Model file for the job. Use its own axes, mm. Round coordinates to 2 decimals unless told otherwise and drop trailing zeros. Order: outer loops, then holes, each group sorted by start corner. A loop starts at its lowest first (then second) coordinate and runs counter-clockwise, first axis right, second up. Notation, with made-up numbers: (30.25, -38.5) - (74.25, -38.5) arc R5 ccw to (74.25, -30.5) - close; hole circle Ø8 at (62, 65.5). An arc over 180 degrees is marked (long way). Use one line per item in the form item = value.
from build123d import *

# Parameters (mm, degrees)
F0_W     = 20
F0_H     = 20
F1_DEPTH = 4


with BuildPart() as f1:
    # F0 (on Top) → F1 (new body)
    with BuildSketch(Plane.XY):
        Polygon((-83.155292, 58.819239), (-95, 0), (-95, -50), (-53.394669, -87.909631), (0, -97.459667), (53.394669, -87.909631), (95, -50), (95, 0), (83.155292, 58.819239), (10, 212.371753), (-10, 212.371753), align=None)
        with BuildLine():
            Line((-55, -20), (-55, 17.5))
            Line((-55, 17.5), (-35, 17.5))
            Line((-35, 17.5), (-35, -6))
            Line((-35, -6), (-29, -6))
            ThreePointArc((-29, -6), (-27.585786, -6.585786), (-27, -8))
            ThreePointArc((-27, -8), (-27.585786, -9.414214), (-29, -10))
            Line((-29, -10), (-35, -10))
            Line((-35, -10), (-35, -20))
            Line((-35, -20), (-55, -20))
        make_face(mode=Mode.SUBTRACT)
        with BuildLine():
            Line((35, -6), (35, 17.5))
            Line((35, 17.5), (55, 17.5))
            Line((55, 17.5), (55, -20))
            Line((55, -20), (35, -20))
            Line((35, -20), (35, -10))
            Line((35, -10), (29, -10))
            ThreePointArc((29, -10), (27, -8), (29, -6))
            Line((29, -6), (35, -6))
        make_face(mode=Mode.SUBTRACT)
        with Locations((0, 182.317775)):
            Rectangle(F0_W, F0_H, mode=Mode.SUBTRACT)
    extrude(amount=F1_DEPTH)


solid = f1.part
(1) Slice it at C-C on x = -5. Give the cut face in (y, z).
Report:
outline = (-96.57, 0) - (172.32, 0) - (172.32, 4) - (-96.57, 4) - close; (192.32, 0) - (212.37, 0) - (212.37, 4) - (192.32, 4) - close
(2) Slice it at B-B on y = 7.5. Give the cut face in (x, z).
Report:
outline = (-93.49, 0) - (-55, 0) - (-55, 4) - (-93.49, 4) - close; (-35, 0) - (35, 0) - (35, 4) - (-35, 4) - close; (55, 0) - (93.49, 0) - (93.49, 4) - (55, 4) - close
(3) Slice it at D-D on y = 54.5. Give the cut face in (x, z).
Report:
outline = (-84.03, 0) - (84.03, 0) - (84.03, 4) - (-84.03, 4) - close
(4) Pull direction Z, two halves, no side cores. Call faces 1 (the face through (-1, 25, 4)), 2 (the face through (-27.07, -92.62, 1.97)), 3 (the face through (-1, 25, 0)): released by +Z, released by -Z, zero draft, split by the parting line, or undercut.
Report:
face_1 = released by +Z
face_2 = zero draft
face_3 = released by -Z
(5) Probe probe 1 along X at (y, z) = (-15, 2.8); probe 2 along X at (y, z) = (174, 3); probe 3 along Y at (x, z) = (4.5, 3.45). List the from-to ranges inside material, lowest first. Write a range as [from, to].
Report:
probe_1 = [-95, -55], [-35, 35], [55, 95]
probe_2 = [-28.28, -10], [10, 28.28]
probe_3 = [-96.65, 172.32], [192.32, 212.37]
(6) Slice it at A-A on z = 3.4. Count the separate pieces of the cut face and the enclosed holes in it, then the cut area to 3 significant figures.
Report:
separate_pieces = 1
enclosed_holes = 3
area = 38,500 mm2
(7) Pin check, flat tips, straight feed: pin 1 (2 mm diameter, centred on x = 62, z = 3, fed in from +Y); pin 2 (1.2 mm diameter, centred on y = 2.5, z = 2, fed in from -X); pin 3 (1.5 mm diameter, centred on x = 11.5, z = 2, fed in from +Y). Stop position of each tip, or through.
Report:
pin_1 = 105.32
pin_2 = -94.62
pin_3 = 210.8
